Check sheet for the modelled part. Datum: model origin and axes. Units: mm. Face numbers are marked on the shaded views. A direction names the side the tool comes from. Give positions to 0.01 mm unless a question says otherwise; leave off trailing zeros. Write each loop counter-clockwise with the first axis right and the second up, starting at its lowest first coordinate (ties: lowest second). Pieces come first, ordered by that corner, then holes. Notation, with made-up numbers: (24, 36.5) -> (66, 36.5) arc R24 cw to (66, 64.5) -> close; hole circle Ø10 at (53.25, 42). An arc over 180 degrees is marked (long way). Use a Markdown table: item, result. Add a question column.
1. Scan lines: probe 1 along Z at (x, y) = (-56.95, 25); probe 2 along Z at (x, y) = (-41, 47); probe 3 along X at (y, z) = (37, 51.5). Record each from-to range of solid material in increasing order. Write a range as [from, to].
2. Cross-section at B-B (x = -38.5). Enter the section's corners in (y, z), then the cut area to 3 significant figures.
3. Cross-section at D-D (y = 10). Enter the section's corners in (x, z), then the cut area to 3 significant figures.
4. Gauge pin test, flat ends, axial feed: P1, Ø3, axis at x = -12, y = 5, coming from the +Z side; P2, Ø20, axis at y = 25, z = 57.79, coming from the -X side; P3, Ø10, axis at y = 19.5, z = 46.5, coming from the +X side. Record the tip position at first contact, or that the pin passes through.
5. Cross-section at C-C (z = 67). Enter the section's corners in (x, y), then the cut area to 3 significant figures.
6. Cross-section at A-A (y = 25). Enter the section's corners in (x, z).
7. Set-up check for the marked faces 1 and 2: record each of +Z, -Z, +X, -X, +Y, -Y from which the full face is reachable in a straight line by a thin tool's end or side.
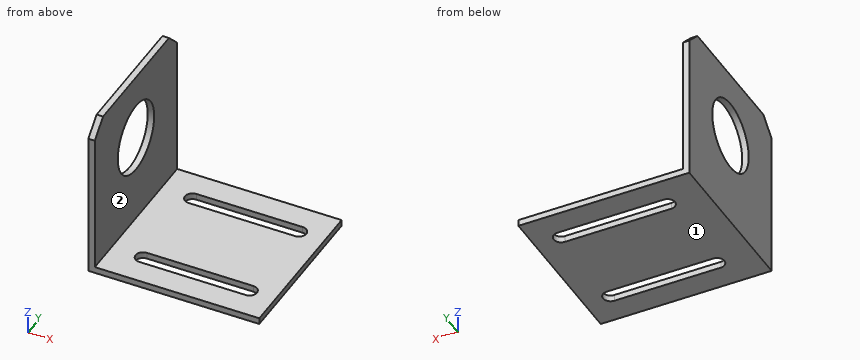
from build123d import *

# Parameters (mm, degrees)
F1_DEPTH = 50
F2_R     = 11.05
F3_DEPTH = 2
F5_DEPTH = 2


with BuildPart() as f1:
    # F0 (on Front) → F1 (new body)
    with BuildSketch(Plane.XZ):
        Polygon((-56.332381, 78.789798), (-58.332381, 78.789798), (-58.332381, 27.789798), (-5.332381, 27.789798), (-5.332381, 29.789798), (-56.332381, 29.789798), align=None)
    extrude(amount=-F1_DEPTH)

    # F2 (on face) → F3 (cut)
    with BuildSketch(Plane.YZ.offset(-56.332381)):
        with Locations((25, 57.789798)):
            Circle(F2_R)
        Polygon((0, 78.789798), (0, 73.789798), (5, 78.789798), align=None)
        Polygon((50, 78.789798), (45, 78.789798), (50, 73.789798), align=None)
    extrude(amount=-F3_DEPTH, mode=Mode.SUBTRACT)

    # F4 (on face) → F5 (cut)
    with BuildSketch(Plane.XY.offset(29.789798)):
        with BuildLine():
            ThreePointArc((-46.481331, 12.310056), (-48.791387, 10), (-46.481331, 7.689944))
            Line((-46.481331, 7.689944), (-13.480531, 7.689944))
            ThreePointArc((-13.480531, 7.689944), (-11.170475, 10), (-13.480531, 12.310056))
            Line((-13.480531, 12.310056), (-46.481331, 12.310056))
        make_face()
        with BuildLine():
            ThreePointArc((-46.481331, 42.310056), (-48.791387, 40), (-46.481331, 37.689944))
            Line((-46.481331, 37.689944), (-13.480531, 37.689944))
            ThreePointArc((-13.480531, 37.689944), (-11.170475, 40), (-13.480531, 42.310056))
            Line((-13.480531, 42.310056), (-46.481331, 42.310056))
        make_face()
    extrude(amount=-F5_DEPTH, mode=Mode.SUBTRACT)


solid = f1.part
Worked answers:
| question | item | result |
|---|---|---|
| 1 | probe 1 | z = [27.79, 46.74], [68.84, 78.79] |
| 1 | probe 2 | z = [27.79, 29.79] |
| 1 | probe 3 | x = [-58.33, -56.33] |
| 2 | outline | (0, 27.79) -> (7.69, 27.79) -> (7.69, 29.79) -> (0, 29.79) -> close; (12.31, 27.79) -> (37.69, 27.79) -> (37.69, 29.79) -> (12.31, 29.79) -> close; (42.31, 27.79) -> (50, 27.79) -> (50, 29.79) -> (42.31, 29.79) -> close |
| 2 | area | 81.5 mm² |
| 3 | outline | (-58.33, 27.79) -> (-48.79, 27.79) -> (-48.79, 29.79) -> (-56.33, 29.79) -> (-56.33, 78.79) -> (-58.33, 78.79) -> close; (-11.17, 27.79) -> (-5.33, 27.79) -> (-5.33, 29.79) -> (-11.17, 29.79) -> close |
| 3 | area | 129 mm² |
| 4 | P1 | stops at z = 29.79 |
| 4 | P2 | passes through |
| 4 | P3 | stops at x = -56.33 |
| 5 | outline | (-58.33, 0) -> (-56.33, 0) -> (-56.33, 18.89) -> (-58.33, 18.89) -> close; (-58.33, 31.11) -> (-56.33, 31.11) -> (-56.33, 50) -> (-58.33, 50) -> close |
| 5 | area | 75.6 mm² |
| 6 | outline | (-58.33, 27.79) -> (-5.33, 27.79) -> (-5.33, 29.79) -> (-56.33, 29.79) -> (-56.33, 46.74) -> (-58.33, 46.74) -> close; (-58.33, 68.84) -> (-56.33, 68.84) -> (-56.33, 78.79) -> (-58.33, 78.79) -> close |
| 7 | face 1 | -Z, +X, -X, +Y, -Y |
| 7 | face 2 | +Z, +X, +Y, -Y |
